The listing builds one solid part. Answer for the finished solid, in the listing's coordinates (mm). A direction names the side the tool comes from. Give positions to 0.01 mm unless a question says otherwise; leave off trailing zeros. Order: outer loops, then holes, each group sorted by start corner. A loop starts at its lowest first (then second) coordinate and runs counter-clockwise, first axis right, second up. Notation, with made-up numbers: M -24,54.25 L -14,54.25 A19 ccw -14,75.25 Z; hole C -18,48.5 d9. An arc over 180 degrees is marked long. Answer as a JSON object with one key per item and string values. Group by question number.
```python
from build123d import *

# Parameters (mm, degrees)
F0_W      = 120
F0_H      = 70
F0_H_2    = 5
F0_H_3    = 125
F1_DEPTH  = 50
F2_DEPTH  = 50
F3_W      = 190
F3_H      = 90
F4_DEPTH  = 100
F5_R      = 31
F6_DEPTH  = 25
F7_R      = 5
F8_DEPTH  = 25
F9_DEPTH  = 50
F10_DEPTH = 50
F11_R     = 5
F12_DEPTH = 25


with BuildPart() as f1:
    # F0 (on Top) → F1 (new body)
    with BuildSketch(Plane.XY):
        with Locations((0, 65)):
            Rectangle(F0_W, F0_H)
        with Locations((0, 27.5)):
            Rectangle(F0_W, F0_H_2)
        with Locations((0, -37.5)):
            Rectangle(F0_W, F0_H_3)
    extrude(amount=-F1_DEPTH)

    # F0 (on Top) → F2 (join)
    with BuildSketch(Plane.XY):
        with Locations((0, 65)):
            Rectangle(F0_W, F0_H)
        with Locations((0, 27.5)):
            Rectangle(F0_W, F0_H_2)
        with Locations((0, -37.5)):
            Rectangle(F0_W, F0_H_3)
    extrude(amount=F2_DEPTH)

    # F3 (on face) → F4 (cut)
    with BuildSketch(Plane.YZ.offset(60)):
        Rectangle(F3_W, F3_H)
    extrude(amount=-F4_DEPTH, mode=Mode.SUBTRACT)

    # F5 (on face) → F6 (cut)
    with BuildSketch(Plane.XY.offset(50)):
        with Locations((0, 64)):
            Circle(F5_R)
    extrude(amount=-F6_DEPTH, mode=Mode.SUBTRACT)

    # F7 (on face) → F8 (cut)
    with BuildSketch(Plane(origin=(0, 100, 0), x_dir=(-1, 0, 0), z_dir=(0, 1, 0))):
        Circle(F7_R)
    extrude(amount=-F8_DEPTH, mode=Mode.SUBTRACT)

    # F0 (on Top) → F9 (join)
    with BuildSketch(Plane.XY):
        with Locations((0, 27.5)):
            Rectangle(F0_W, F0_H_2)
    extrude(amount=F9_DEPTH)

    # F0 (on Top) → F10 (join)
    with BuildSketch(Plane.XY):
        with Locations((0, 27.5)):
            Rectangle(F0_W, F0_H_2)
    extrude(amount=-F10_DEPTH)

    # F11 (on face) → F12 (cut)
    with BuildSketch(Plane.XZ.offset(-25)):
        Circle(F11_R)
    extrude(amount=-F12_DEPTH, mode=Mode.SUBTRACT)


solid = f1.part
```
Item 1: A tool of negligible diameter and unlimited length cuts with its end or side. For faces 1 (the flat face through (11, 62, -45)), 2 (the flat face through (-1, 100, -12)), 3 (the cylindrical face through (-4.036, 94.736, 47.535)), from which of +Z, -Z, +X, -X, +Y, -Y can it reach the whole face along a straight path? Write none if from no direction.
Item 2: Section C-C (y = -54.5) is taken. Determine the outline of the cut face in (x, z).
Item 3: Determine the mould class of faces 4 (the cylindrical face through (-1.08, 27.46, -4.88)), 5 (the flat face through (-40, -36, 1)), 6 (the flat face through (-60, -1, 1)), 7 (the flat face through (-1, 1, -50)) for opening direction X: released by +X, released by -X, zero draft, split by the parting line, or undercut.
Item 4: Consider probe 1 along Y at (x, z) = (-22.5, -36); probe 2 along Y at (x, z) = (0, 46.8); probe 3 along Z at (x, y) = (0, 27.2). Determine where each line is inside the solid, lowest interval first. Write a range as from..to.
Item 5: Section D-D (z = 17.5) is taken. Determine the outline of the cut face in (x, y), and give its area (3 significant figures).
Item 6: Section B-B (z = 0) is taken. Determine the outline of the cut face in (x, y), and give its area (3 significant figures).
Item 7: Section A-A (x = -34) is taken. Determine the outline of the cut face in (y, z), and give its area (3 significant figures).
Item 8: Flat-ended cylindrical pins translate along their axes: P1, Ø9, axis at x = 0, z = 0, coming from the +Y side; P2, Ø10, axis at y = -30.5, z = 23, coming from the +X side. Find the tip coordinate at first contact, or state that the pin passes through.
Values found:
{
 "1": {"face 1": "+X", "face 2": "+Z, -Z, +X, -X, +Y", "face 3": "+Z"},
 "2": {"outline": "M -60,-50 L 60,-50 L 60,-45 L -40,-45 L -40,45 L 60,45 L 60,50 L -60,50 Z"},
 "3": {"face 4": "undercut", "face 5": "released by +X", "face 6": "released by -X", "face 7": "zero draft"},
 "4": {"probe 1": "y = -100..-95, 25..30, 95..100", "probe 2": "y = -100..33, 95..100", "probe 3": "z = -50..-5, 5..50"},
 "5": {"outline": "M -60,-100 L 60,-100 L 60,-95 L -40,-95 L -40,25 L 60,25 L 60,30 L -40,30 L -40,95 L 60,95 L 60,100 L -60,100 Z", "area": "5,500 mm^2"},
 "6": {"outline": "M -60,-100 L 60,-100 L 60,-95 L -40,-95 L -40,25 L -5,25 L -5,30 L -40,30 L -40,95 L -5,95 L -5,100 L -60,100 Z; M 5,25 L 60,25 L 60,30 L 5,30 Z; M 5,95 L 60,95 L 60,100 L 5,100 Z", "area": "5,400 mm^2"},
 "7": {"outline": "M -100,-50 L 100,-50 L 100,50 L -100,50 Z; hole M -95,-45 L 25,-45 L 25,45 L -95,45 Z; hole M 30,-45 L 95,-45 L 95,45 L 30,45 Z", "area": "3,350 mm^2"},
 "8": {"P1": "stops at y = -95", "P2": "stops at x = -40"}
}
